Source: three-view drawing plus pictorial views. Frame: mm from the lowest corner of the part. A direction names the side the tool comes from. Coordinates: 2 decimals unless noted, no trailing zeros. Write each loop counter-clockwise with the first axis right and the second up, starting at its lowest first coordinate (ties: lowest second). Pieces come first, ordered by that corner, then holes. Notation, with made-up numbers: (-22.5, -5) -> (-8.5, -5) arc R23 cw to (-8.5, 10) -> close; hole circle Ø9 at (43.25, -36). An arc over 180 degrees is marked (long way). One line per item, written item: value.
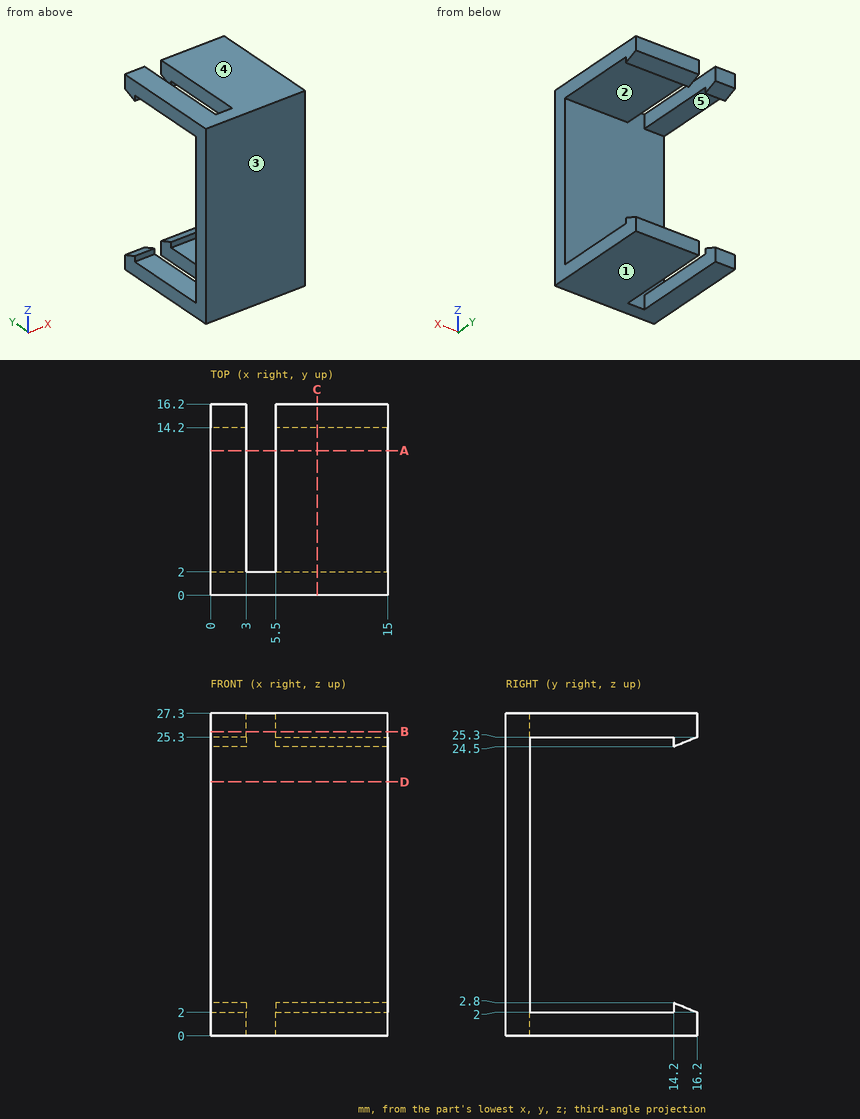
(1) Section A-A (y = 12.25). Return the cut outline in (x, z).
Responses:
outline: (0, 0) -> (3, 0) -> (3, 2) -> (0, 2) -> close; (0, 25.3) -> (3, 25.3) -> (3, 27.3) -> (0, 27.3) -> close; (5.5, 0) -> (15, 0) -> (15, 2) -> (5.5, 2) -> close; (5.5, 25.3) -> (15, 25.3) -> (15, 27.3) -> (5.5, 27.3) -> close
(2) Pull-direction query (Z, two-part tool) for the marked faces 1, 2 and 3; classes: released by +Z, released by -Z, zero draft, split by the parting line, or undercut.
Responses:
face 1: released by -Z
face 2: undercut
face 3: zero draft
(3) Section B-B (z = 25.75). Return the cut outline in (x, y), then the cut area to 4 significant figures.
Responses:
outline: (0, 0) -> (15, 0) -> (15, 16.2) -> (5.5, 16.2) -> (5.5, 2) -> (3, 2) -> (3, 16.2) -> (0, 16.2) -> close
area: 207.5 mm2
(4) Section C-C (x = 9). Return the cut outline in (y, z), then the cut area to 3 significant figures.
Responses:
outline: (0, 0) -> (16.2, 0) -> (16.2, 2) -> (14.2, 2.8) -> (14.2, 2) -> (2, 2) -> (2, 25.3) -> (14.2, 25.3) -> (14.2, 24.5) -> (16.2, 25.3) -> (16.2, 27.3) -> (0, 27.3) -> close
area: 113 mm2
(5) Section D-D (z = 21.5). Return the cut outline in (x, y).
Responses:
outline: (0, 0) -> (15, 0) -> (15, 2) -> (0, 2) -> close
(6) Reachability of the marked faces 4 and 5 from +Z, -Z, +X, -X, +Y, -Y: full face, straight path, thin tool, end or side. Return the list, or none.
Responses:
face 4: +Z, +X, -X, +Y, -Y
face 5: +X, -X
(7) First-contact query: pin 1 (0.6 mm diameter, centred on x = 1.5, z = 25, fed in from -Y); pin 2 (8 mm diameter, centred on x = 2.5, z = 7.5, fed in from +Y). Flat tips, straight axial feed; report the tip coordinate or a pass-through.
Responses:
pin 1: stops at y = 0
pin 2: stops at y = 2
(8) Line query: line 1 (Z direction, x = 11.5, y = 3); line 2 (X direction, y = 14, z = 26.25); line 3 (Y direction, x = 9.75, z = 21.75). Output: solid intervals per line, ascending. Write a range as [from, to].
Responses:
line 1: z = [0, 2], [25.3, 27.3]
line 2: x = [0, 3], [5.5, 15]
line 3: y = [0, 2]
